```python
from build123d import *

# Parameters (mm, degrees)
BASPROSKE_W        = 8
BASPROSKE_H        = 9
TOOTHCUT_DEPTH     = 16.033296378
TEETHCUTS_COUNT    = 10
TEETHCUTS_ANGLE    = 324
BORSKE_R           = 1.5
BORE_DEPTH         = 50.0000508
SKETCH2_R          = 1.6
CUT_EXTRUDE1_DEPTH = 10


with BuildPart() as part:
    # BasProSke → Base-Revolve (revolve)
    with BuildSketch(Plane(origin=(0, 0, 0), x_dir=(1, 0, 0), z_dir=(0, 1, 0)), mode=Mode.PRIVATE) as base_revolve_sk:
        with Locations((4, 4.5)):
            Rectangle(BASPROSKE_W, BASPROSKE_H)
    revolve(base_revolve_sk.sketch.rotate(Axis((-10, 0, 0), (1, 0, 0)), 180), axis=Axis((-10, 0, 0), (1, 0, 0)))

    # TooCutSke → ToothCut (cut, through all)
    with BuildSketch(Plane(origin=(0, 0, 0), x_dir=(0, 0, -1), z_dir=(1, 0, 0))):
        with BuildLine():
            ThreePointArc((0.883878355, 5.554109745), (0, 5.624), (-0.883878355, 5.554109745))
            ThreePointArc((-0.883878355, 5.554109745), (-1.258245767, 7.379188248), (-2.637816971, 8.631324741))
            ThreePointArc((-2.637816971, 8.631324741), (0, 9.0254), (2.637816971, 8.631324741))
            ThreePointArc((2.637816971, 8.631324741), (1.258245767, 7.379188248), (0.883878355, 5.554109745))
        make_face()
    toothcut = extrude(amount=TOOTHCUT_DEPTH, mode=Mode.SUBTRACT)

    # TeethCuts: ToothCut ×10 about axis
    teethcuts_axis = Axis((-10, 0, 0), (1, 0, 0))
    for i in range(1, TEETHCUTS_COUNT):
        add(toothcut.rotate(teethcuts_axis, i * TEETHCUTS_ANGLE / (TEETHCUTS_COUNT - 1)), mode=Mode.SUBTRACT)

    # BorSke → Bore (cut, symmetric)
    with BuildSketch(Plane(origin=(0, 0, 0), x_dir=(0, 0, -1), z_dir=(1, 0, 0))):
        with Locations(Location((0, 0, 0), (0, 0, 180))):
            Circle(BORSKE_R)
    extrude(amount=BORE_DEPTH, both=True, mode=Mode.SUBTRACT)

    # Sketch1 → Cut-Revolve1 (revolve, cut)
    with BuildSketch(Plane(origin=(0, 0, 0), x_dir=(1, 0, 0), z_dir=(0, 1, 0)), mode=Mode.PRIVATE) as cut_revolve1_sk:
        Polygon((0, -5), (3.946553979, -11.835632006), (4.053446021, -11.835632006), (8, -5), (10.092806182, -15.908435196), (-2.21285392, -14.524958616), align=None)
    revolve(cut_revolve1_sk.sketch.rotate(Axis((0, 0, 0), (-1, 0, 0)), 180), axis=Axis((0, 0, 0), (-1, 0, 0)), mode=Mode.SUBTRACT)

    # Sketch2 → Cut-Extrude1 (cut)
    with BuildSketch(Plane.ZY):
        Circle(SKETCH2_R)
    extrude(amount=-CUT_EXTRUDE1_DEPTH, mode=Mode.SUBTRACT)


solid = part.part
```
Work out the finished part from the listing and answer in its coordinate system (mm). Give positions to 0.01 mm unless a question says otherwise; leave off trailing zeros. Loops run counter-clockwise (first coordinate to the right, second up) from the corner with the lowest first, then second, coordinate; pieces in that order, holes last. Notation, with made-up numbers: (60, 11.5) -> (91, 11.5) arc R23 cw to (91, 20.5) -> close; hole circle Ø11 at (-18, 38.5). An arc over 180 degrees is marked (long way). Put each result on its own line as item: value. Start each with the question number.
Item 1: The part is cut by section A-A (z = 0). Give the vertices of the cut face in (x, y).
Item 2: Find the intervals of material crossed by L1, parallel to Y at x = 4.75, z = 2.75; L2, parallel to Y at x = 6, z = 0; L3, parallel to Y at x = 2.25, z = 3, in increasing order. Write a range as [from, to].
Item 3: Each of these flat-tipped pins is pushed along its axis until it touches: P1, Ø1, axis at x = 2, z = -3.5, coming from the +Y side; P2, Ø1, axis at x = 2, z = 4, coming from the -Y side; P3, Ø2, axis at x = 7, z = 4.5, coming from the +Y side. Where does it stop, or does it pass through?
Item 4: The mould has two halves that part along Z. Classify faces 1 (the face through (8, 0, -2)), 2 (the face through (3.949, -6.256, 3.233)): released by +Z, released by -Z, zero draft, split by the parting line, or undercut.
Answers below:
1. outline: (0, -5) -> (0.36, -5.62) -> (7.64, -5.62) -> (8, -5) -> (8, -1.6) -> (0, -1.6) -> close; (0, 1.6) -> (8, 1.6) -> (8, 5) -> (7.64, 5.62) -> (0.36, 5.62) -> (0, 5) -> close
2. L1: [-8.57, -5.26], [-4.91, 4.91], [5.26, 8.57]
2. L2: [-5.62, -1.6], [1.6, 5.62]
2. L3: [-8.38, -5.66], [-4.76, 4.76], [5.66, 8.38]
3. P1: y = 8.31
3. P2: y = -4.65
3. P3: y = 5.25
4. face 1: zero draft
4. face 2: undercut
